Could you check a few things on this drawing? It's one solid part, dimensions in mm from its lowest x, y, z. A direction names the side the tool comes from. Coordinates: 2 decimals unless noted, no trailing zeros. Write each loop counter-clockwise with the first axis right and the second up, starting at its lowest first coordinate (ties: lowest second). Pieces come first, ordered by that corner, then holes. Notation, with made-up numbers: M 62.25,44.25 L 88.25,44.25 A35 cw 88.25,77.25 Z; hole C -20.75,32 d11. An arc over 180 degrees is marked long. Use a Markdown table: item, result.
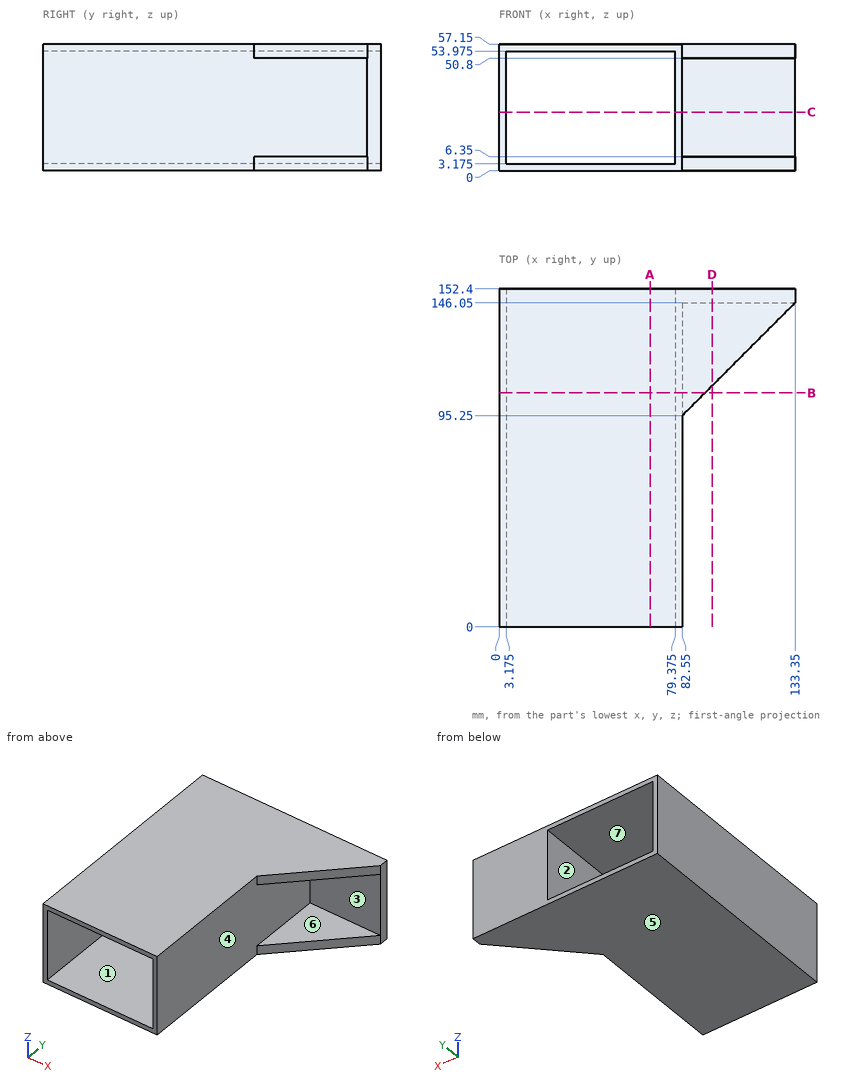
1. Suppose I cut it at C-C on z = 26.5. Write out the boundary of the cut face in (x, y) (3 decimals).
Answers follow:
| item | result |
|---|---|
| outline | M 0,0 L 3.175,0 L 3.175,152.4 L 0,152.4 Z; M 79.375,0 L 82.55,0 L 82.55,146.05 L 133.35,146.05 L 133.35,152.4 L 79.375,152.4 Z |
2. Which directions (+Z, -Z, +X, -X, +Y, -Y) give clear straight access to the entire face, cutting with the end or side of a thin tool? Please do the marked faces 5, 6 and 7.
Answers follow:
| item | result |
|---|---|
| face 5 | -Z, +X, -X, +Y, -Y |
| face 6 | +X, -Y |
| face 7 | +Y, -Y |
3. I need wall thicknesses on probe 1 along X at (y, z) = (134.5, 13) (3 decimals); probe 2 along Z at (x, y) = (8, 139) (3 decimals); probe 3 along Z at (x, y) = (123.5, 145). Which ranges of each line are inside material? Lowest first, please.
Answers follow:
| item | result |
|---|---|
| probe 1 | x = 0 to 3.175, 79.375 to 82.55 |
| probe 2 | z = 0 to 3.175, 53.975 to 57.15 |
| probe 3 | z = 0 to 6.35, 50.8 to 57.15 |
4. Suppose I cut it at D-D on x = 96. Write out the boundary of the cut face in (y, z), and give its area (3 significant figures).
Answers follow:
| item | result |
|---|---|
| outline | M 108.7,0 L 152.4,0 L 152.4,57.15 L 108.7,57.15 L 108.7,50.8 L 146.05,50.8 L 146.05,6.35 L 108.7,6.35 Z |
| area | 837 mm2 |
5. Suppose I cut it at B-B on y = 105.5. Write out the boundary of the cut face in (x, z) (3 decimals).
Answers follow:
| item | result |
|---|---|
| outline | M 0,0 L 92.8,0 L 92.8,6.35 L 82.55,6.35 L 82.55,50.8 L 92.8,50.8 L 92.8,57.15 L 0,57.15 Z; hole M 3.175,3.175 L 79.375,3.175 L 79.375,53.975 L 3.175,53.975 Z |
6. Will this pin go through, and if not, where does the flat tip stop? pin 1 Ø1.5 at (y, z) = (75.5, 14) entering from +X.
Answers follow:
| item | result |
|---|---|
| pin 1 | stops at x = 82.55 |
7. Suppose I cut it at A-A on x = 68. Write out the boundary of the cut face in (y, z) (3 decimals), and give its area (3 significant figures).
Answers follow:
| item | result |
|---|---|
| outline | M 0,0 L 152.4,0 L 152.4,3.175 L 0,3.175 Z; M 0,53.975 L 152.4,53.975 L 152.4,57.15 L 0,57.15 Z |
| area | 968 mm2 |
8. We'd pull the mould along X, two halves only. Please class the marked faces 1, 2, 3 and 4: +X half, -X half, draft (parallel to the pull), parting line (faces both ways), or undercut.
Answers follow:
| item | result |
|---|---|
| face 1 | undercut |
| face 2 | undercut |
| face 3 | draft |
| face 4 | +X half |
